from build123d import *

# Parameters (mm, degrees)
F0_W     = 150
F0_H     = 100
F1_DEPTH = 16
F2_R     = 5
F3_DEPTH = 15
F4_W     = 130
F4_H     = 35.7704423368
F5_DEPTH = 10
F6_R     = 2.8732308489
F7_DEPTH = 7
F8_W     = 2
F8_H     = 10.8852211684
F8_H_2   = 14
F9_DEPTH = 35


with BuildPart() as f1:
    # F0 (on Front) → F1 (new body)
    with BuildSketch(Plane.XZ):
        with Locations((-201.6328409241, 45.7894764841)):
            Rectangle(F0_W, F0_H)
    extrude(amount=F1_DEPTH)

    # F2 (on face) → F3 (join)
    with BuildSketch(Plane.XZ.offset(16)):
        with Locations((-136.6328409241, 85.7894764841)):
            Circle(F2_R)
        with Locations((-136.6328409241, 5.7894764841)):
            Circle(F2_R)
    extrude(amount=F3_DEPTH)

    # F4 (on face) → F5 (cut)
    with BuildSketch(Plane.XZ.offset(16)):
        with Locations((-191.6328409241, 45.7894764841)):
            Rectangle(F4_W, F4_H)
    extrude(amount=-F5_DEPTH, mode=Mode.SUBTRACT)

    # F6 (on face) → F7 (cut)
    with BuildSketch(Plane.XZ.offset(6)):
        with Locations((-145.006071773, 45.7894764841)):
            Circle(F6_R)
        with BuildLine():
            Line((-126.6328409241, 38.7894764841), (-126.6328409241, 52.7894764841))
            ThreePointArc((-126.6328409241, 52.7894764841), (-133.6328409241, 45.7894764841), (-126.6328409241, 38.7894764841))
        make_face()
        with BuildLine():
            ThreePointArc((-126.6328409241, 38.7894764841), (-121.6830934558, 40.8397290158), (-119.6328409241, 45.7894764841))
            ThreePointArc((-119.6328409241, 45.7894764841), (-121.6830934558, 50.7392239524), (-126.6328409241, 52.7894764841))
            Line((-126.6328409241, 52.7894764841), (-126.6328409241, 38.7894764841))
        make_face()
    extrude(amount=-F7_DEPTH, mode=Mode.SUBTRACT)

    # F8 (on face) → F9 (cut)
    with BuildSketch(Plane.YZ.offset(-126.6328409241)):
        with Locations((-3, 33.3468658999)):
            Rectangle(F8_W, F8_H)
        with Locations((-3, 45.7894764841)):
            Rectangle(F8_W, F8_H_2)
        with Locations((-3, 58.2320870683)):
            Rectangle(F8_W, F8_H)
    extrude(amount=-F9_DEPTH, mode=Mode.SUBTRACT)


solid = f1.part
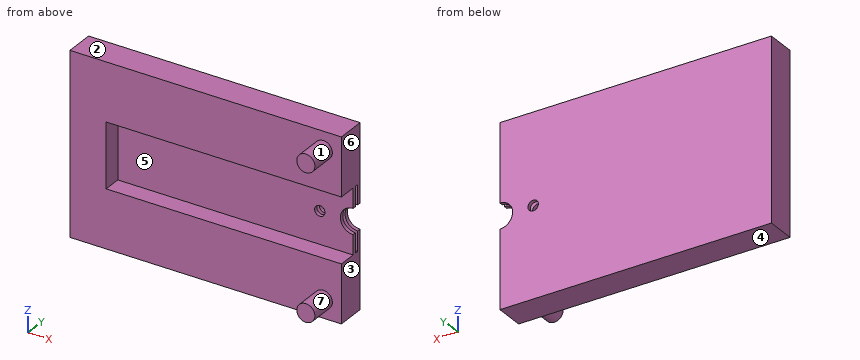
Check sheet for the modelled part. Datum: model origin and axes. Units: mm. Face numbers are marked on the shaded views. A direction names the side the tool comes from. Round coordinates to 2 decimals unless told otherwise and drop trailing zeros. Loops run counter-clockwise (first coordinate to the right, second up) from the corner with the lowest first, then second, coordinate; pieces in that order, holes last. Notation, with made-up numbers: (77.5, 59.25) -> (112.5, 59.25) arc R24 ccw to (112.5, 73.25) -> close; hole circle Ø1 at (41.25, 2.5). An arc over 180 degrees is marked (long way). Put each result on its own line as item: value. Start each with the question number.
1. Section check B-B (z = 33.5). Enter the section's corners in (x, y), plus the area to 3 significant figures.
2. Section check C-C (y = -9.5). Enter the section's corners in (x, z), plus the area to 3 significant figures.
3. Scan lines: probe 1 along Y at (x, z) = (-148, 61.5); probe 2 along Z at (x, y) = (-182, -15); probe 3 along Y at (x, z) = (-248.5, 10). Record each from-to range of solid material in increasing order.
4. Access from +Z, -Z, +X, -X, +Y, -Y to the whole of each face (thin tool, end or side, straight path). Record for the marked faces 5, 6 and 7.
5. Draft check along Z on the marked faces 1, 2, 3 and 4. Enter one of: +Z half, -Z half, draft (parallel to the pull), parting line (faces both ways), or undercut.
6. Gauge pin test, flat ends, axial feed: pin 1 (1 mm diameter, centred on x = -244.5, z = 63.5, fed in from -Y); pin 2 (7.5 mm diameter, centred on x = -145.01, z = 45.79, fed in from -Y); pin 3 (11 mm diameter, centred on y = -12, z = 38, fed in from +X). Record the tip position at first contact, or that the pin passes through.
7. Section check D-D (x = -168). Enter the section's corners in (y, z).
8. Section check A-A (x = -146). Enter the section's corners in (y, z).
Findings:
1. outline: (-276.63, -16) -> (-256.63, -16) -> (-256.63, -6) -> (-126.63, -6) -> (-126.63, -4) -> (-161.63, -4) -> (-161.63, -2) -> (-126.63, -2) -> (-126.63, 0) -> (-276.63, 0) -> close
1. area: 1,030 mm^2
2. outline: (-276.63, -4.21) -> (-126.63, -4.21) -> (-126.63, 27.9) -> (-256.63, 27.9) -> (-256.63, 63.67) -> (-126.63, 63.67) -> (-126.63, 95.79) -> (-276.63, 95.79) -> close
2. area: 10,300 mm^2
3. probe 1: y = -6 to -4, -2 to 0
3. probe 2: z = -4.21 to 27.9, 63.67 to 95.79
3. probe 3: y = -16 to 0
4. face 5: +X, -Y
4. face 6: +Z, -Z, +X, +Y, -Y
4. face 7: -Y
5. face 1: undercut
5. face 2: +Z half
5. face 3: draft
5. face 4: -Z half
6. pin 1: stops at y = -16
6. pin 2: stops at y = -6
6. pin 3: stops at x = -256.63
7. outline: (-16, -4.21) -> (0, -4.21) -> (0, 95.79) -> (-16, 95.79) -> (-16, 63.67) -> (-6, 63.67) -> (-6, 27.9) -> (-16, 27.9) -> close
8. outline: (-16, -4.21) -> (0, -4.21) -> (0, 43.09) -> (-2, 43.09) -> (-2, 27.9) -> (-4, 27.9) -> (-4, 43.09) -> (-6, 43.09) -> (-6, 27.9) -> (-16, 27.9) -> close; (-16, 63.67) -> (-6, 63.67) -> (-6, 48.49) -> (-4, 48.49) -> (-4, 63.67) -> (-2, 63.67) -> (-2, 48.49) -> (0, 48.49) -> (0, 95.79) -> (-16, 95.79) -> close
